Input: part model. Units: mm. Frame: model coordinates. A direction names the side the tool comes from. Coordinates: 2 decimals unless noted, no trailing zeros. Order: outer loops, then holes, each group sorted by start corner. A loop starts at its lowest first (then second) coordinate and runs counter-clockwise, first axis right, second up. Notation, with made-up numbers: (-10, 15) -> (28, 15) arc R25 ccw to (28, 54) -> close; hole circle Ø7 at (87.5, 8). An arc over 180 degrees is marked (long way). Answer as CSV lines item,"result".
from build123d import *

# Parameters (mm, degrees)
SKETCH1_R               = 40
BOSS_EXTRUDE1_DEPTH     = 74.5
SKETCH3_R               = 40
SKETCH3_R_2             = 25
CUT_EXTRUDE1_DEPTH      = 21
CUT_EXTRUDE2_DEPTH      = 22
CUT_EXTRUDE2_DEPTH_BACK = 22
SKETCH2_R               = 40
SKETCH2_R_2             = 37.5
CUT_EXTRUDE4_DEPTH      = 160.376911753
FILLET1_R               = 2
CUT_EXTRUDE5_DEPTH      = 160.376911753
SKETCH8_R               = 3.75
CUT_EXTRUDE6_DEPTH      = 140.942845476
CUT_EXTRUDE7_DEPTH      = 94.542770966
CUT_EXTRUDE8_DEPTH      = 10
FILLET2_R               = 1
FILLET3_R               = 1


with BuildPart() as part:
    # Sketch1 → Boss-Extrude1 (new, symmetric)
    with BuildSketch(Plane(origin=(0, 0, 0), x_dir=(1, 0, 0), z_dir=(0, 1, 0))):
        with Locations(Location((0, 0, 0), (0, 0, 270))):
            Circle(SKETCH1_R)
    extrude(amount=BOSS_EXTRUDE1_DEPTH, both=True)

    # Sketch3 → Cut-Extrude1 (cut)
    with BuildSketch(Plane(origin=(0, 74.5, 0), x_dir=(1, 0, 0), z_dir=(0, 1, 0))):
        with Locations(Location((0, 0, 0), (0, 0, 270))):
            Circle(SKETCH3_R)
        with Locations(Location((0, 0, 0), (0, 0, 270))):
            Circle(SKETCH3_R_2, mode=Mode.SUBTRACT)
    cut_extrude1 = extrude(amount=-CUT_EXTRUDE1_DEPTH, mode=Mode.SUBTRACT)

    # Mirror1: Cut-Extrude1 across plane
    add(cut_extrude1.mirror(Plane.ZX), mode=Mode.SUBTRACT)

    # Sketch2 → Cut-Extrude2 (cut, two sides: drawn at the far end of the back side and taken through both)
    with BuildSketch(Plane(origin=(0, 0, 0), x_dir=(1, 0, 0), z_dir=(0, 1, 0)).offset(-CUT_EXTRUDE2_DEPTH_BACK)):
        with Locations(Location((0, 0, 0), (0, 0, 270))):
            Circle(SKETCH2_R)
        with Locations(Location((0, 0, 0), (0, 0, 90))):
            Circle(SKETCH2_R_2, mode=Mode.SUBTRACT)
    extrude(amount=CUT_EXTRUDE2_DEPTH + CUT_EXTRUDE2_DEPTH_BACK, mode=Mode.SUBTRACT)

    # Sketch5 → Cut-Extrude4 (cut, through all)
    with BuildSketch(Plane(origin=(0, 74.5, 0), x_dir=(1, 0, 0), z_dir=(0, 1, 0))):
        with BuildLine():
            Line((-12, 13), (12, 13))
            ThreePointArc((12, 13), (15, 10), (12, 7))
            Line((12, 7), (-12, 7))
            ThreePointArc((-12, 7), (-15, 10), (-12, 13))
        make_face()
    extrude(amount=-CUT_EXTRUDE4_DEPTH, mode=Mode.SUBTRACT)

    # Fillet1
    fillet1_edges = [part.edges().sort_by_distance(p)[0] for p in [
        (0, -53.5, -25),
        (0, 53.5, -25),
    ]]
    fillet(fillet1_edges, radius=FILLET1_R)

    # Sketch7 → Revolve2 (revolve)
    with BuildSketch(Plane(origin=(0, 0, 0), x_dir=(0, 0, -1), z_dir=(1, 0, 0))):
        Polygon((40, 22), (37.5, 19.5), (37.5, 22), align=None)
    revolve2 = revolve(axis=Axis((0, 103.881416882, 0), (0, -1, 0)))

    # Mirror2: Revolve2 across plane
    add(revolve2.mirror(Plane.ZX))

    # Sketch4 → Cut-Extrude5 (cut, through all)
    with BuildSketch(Plane(origin=(0, 74.5, 0), x_dir=(1, 0, 0), z_dir=(0, 1, 0))):
        with BuildLine():
            Line((0, 0), (0, 40))
            ThreePointArc((0, 40), (28.284271247, 28.284271247), (40, 0))
            Line((40, 0), (0, 0))
        make_face()
    extrude(amount=-CUT_EXTRUDE5_DEPTH, mode=Mode.SUBTRACT)

    # Sketch8 → Cut-Extrude6 (cut, through all)
    with BuildSketch(Plane(origin=(0, 53.5, 0), x_dir=(1, 0, 0), z_dir=(0, 1, 0))):
        with Locations(Location((-8.282209443, 30.909626441, 0), (0, 0, 270))):
            Circle(SKETCH8_R)
        with Locations(Location((30.909626441, -8.282209443, 0), (0, 0, 270))):
            Circle(SKETCH8_R)
        with Locations(Location((22.627416998, -22.627416998, 0), (0, 0, 270))):
            Circle(SKETCH8_R)
        with Locations(Location((8.282209443, -30.909626441, 0), (0, 0, 270))):
            Circle(SKETCH8_R)
        with Locations(Location((-8.282209443, -30.909626441, 0), (0, 0, 270))):
            Circle(SKETCH8_R)
        with Locations(Location((-22.627416998, -22.627416998, 0), (0, 0, 270))):
            Circle(SKETCH8_R)
        with Locations(Location((-30.909626441, -8.282209443, 0), (0, 0, 270))):
            Circle(SKETCH8_R)
        with Locations(Location((-30.909626441, 8.282209443, 0), (0, 0, 270))):
            Circle(SKETCH8_R)
        with Locations(Location((-22.627416998, 22.627416998, 0), (0, 0, 270))):
            Circle(SKETCH8_R)
    extrude(amount=-CUT_EXTRUDE6_DEPTH, mode=Mode.SUBTRACT)

    # Sketch10 → Cut-Extrude7 (cut, through all)
    with BuildSketch(Plane(origin=(0, 0, 0), x_dir=(-1, 0, 0), z_dir=(0, 0, -1))):
        with BuildLine():
            Line((-25.208360839, -42.779227454), (-27.321452148, -47.310766389))
            ThreePointArc((-27.321452148, -47.310766389), (-33.506811582, -45.211119786), (-40, -44.5))
            Line((-40, -44.5), (-40, -53.5))
            Line((-40, -53.5), (-27, -53.5))
            ThreePointArc((-27, -53.5), (-25.585786438, -54.085786438), (-25, -55.5))
            Line((-25, -55.5), (-25, -74.5))
            Line((-25, -74.5), (-10, -74.5))
            ThreePointArc((-10, -74.5), (-10.114159057, -71.885327718), (-10.45576741, -69.29055467))
            Line((-10.45576741, -69.29055467), (-5.531728645, -68.422313782))
            ThreePointArc((-5.531728645, -68.422313782), (-12.23263309, -53.193349985), (-25.208360839, -42.779227454))
        make_face()
    extrude(amount=-CUT_EXTRUDE7_DEPTH, mode=Mode.SUBTRACT)

    # Sketch11 → Cut-Extrude8 (cut)
    with BuildSketch(Plane(origin=(0, 74.5, 0), x_dir=(1, 0, 0), z_dir=(0, 1, 0))):
        with BuildLine():
            Line((-20.784609691, 3), (-4, 3))
            Line((-4, 3), (-4, -4))
            Line((-4, -4), (20.615528128, -4))
            ThreePointArc((20.615528128, -4), (-3.501020872, -20.706106656), (-20.784609691, 3))
        make_face()
    extrude(amount=-CUT_EXTRUDE8_DEPTH, mode=Mode.SUBTRACT)

    # Fillet2
    fillet2_edges = [part.edges().sort_by_distance(p)[0] for p in [
        (20.615528128, 69.5, 4),
        (-20.784609691, 69.5, -3),
        (-4, 69.5, -3),
        (-4, 69.5, 4),
    ]]
    fillet(fillet2_edges, radius=FILLET2_R)

    # Fillet3
    fillet3_edges = [part.edges().sort_by_distance(p)[0] for p in [
        (-3.685711089, 64.5, 20.674030419),
        (-12.449874371, 64.5, -3),
        (8.182458366, 64.5, 4),
        (-4, 64.5, 0.5),
        (20.155486146, 64.5, 4.387627564),
        (-4.292893219, 64.5, -2.707106781),
        (-20.570569135, 64.5, -2.741619849),
        (-3.707106781, 64.5, 3.707106781),
    ]]
    fillet(fillet3_edges, radius=FILLET3_R)


solid = part.part
1. Reachability of faces 5 (the face through (0, 1, -3)), 6 (the face through (-4, 70, 0)), 7 (the face through (-11.943, 0.749, -31.723)) from +Z, -Z, +X, -X, +Y, -Y: full face, straight path, thin tool, end or side. Return the list, or none.
Findings:
face 5,"-Z, +X, +Y, -Y"
face 6,"+Y"
face 7,"+Y, -Y"
2. Cut plane A-A (y = -5). State how many separate pieces and enclosed holes the cut face has, plus the area to 3 significant figures.
Findings:
separate pieces,"1"
enclosed holes,"9"
area,"2,830 mm2"
3. Contact query for flat-ended pins moving along their axis: pin 1 (12 mm diameter, centred on x = 22.63, z = 22.63, fed in from -Y); pin 2 (12 mm diameter, centred on y = -14.5, z = -27, fed in from +X); pin 3 (9.5 mm diameter, centred on x = -4.5, y = 36, fed in from -Z); pin 4 (4 mm diameter, centred on y = 68, z = 1, fed in from -X). Output: stop coordinate, or through.
Findings:
pin 1,"stops at y = -48.45"
pin 2,"stops at x = 0"
pin 3,"stops at z = -40"
pin 4,"stops at x = -25"
4. Mould query, pull axis Z, two halves, no side actions, for faces 1 (the face through (0, 1, -26)), 2 (the face through (-29.78, 0.75, 11.86)), 3 (the face through (-6, 1, -7)), 4 (the face through (-25.711, -19.621, 27.465)). Classes: released by +Z, released by -Z, zero draft, split by the parting line, or undercut.
Findings:
face 1,"zero draft"
face 2,"undercut"
face 3,"undercut"
face 4,"split by the parting line"
5. Cut plane B-B (y = -62.5). Return the cut outline in (x, z), plus the area to 3 significant figures.
Findings:
outline,"(-12, -13) arc R3 cw to (-12, -7) -> (0, -7) -> (0, 0) -> (7.12, 0) -> (7.12, 23.96) arc R25 ccw (long way) to (0, -25) -> (0, -13) -> close"
area,"1,070 mm2"
6. Ray query, line 1 along Z through (x, y) = (-19.5, 22); line 2 along X through (y, z) = (-30.5, 31.5); line 3 along X through (y, z) = (40, 34). Return the intervals inside material, ascending.
Findings:
line 1,"z = -34.92 to -24.7, -20.56 to 20.56, 24.7 to 34.92"
line 2,"x = -24.65 to -11.99, -4.58 to 4.58, 11.99 to 24.65"
line 3,"x = -21.07 to -10.41, -6.16 to 6.16, 10.41 to 21.07"
